from build123d import *

# Parameters (mm, degrees)
SKETCH033_W   = 68
SKETCH033_H   = 36
PAD021_DEPTH  = 1
SKETCH034_W   = 68
SKETCH034_H   = 36
SKETCH034_W_2 = 66
SKETCH034_H_2 = 34
PAD022_DEPTH  = 3
SKETCH036_R   = 1.5
PAD024_DEPTH  = 3
BOX001_W      = 70
BOX001_H      = 38
BOX001_DEPTH  = 5


with BuildPart() as bottommold:
    # Sketch033 → Pad021 (new body)
    with BuildSketch(Plane.XY):
        Rectangle(SKETCH033_W, SKETCH033_H)
    extrude(amount=PAD021_DEPTH)

    # Sketch034 (on Face6 of Pad021) → Pad022 (join)
    with BuildSketch(Plane.XY.offset(1)):
        Rectangle(SKETCH034_W, SKETCH034_H)
        Rectangle(SKETCH034_W_2, SKETCH034_H_2, mode=Mode.SUBTRACT)
    extrude(amount=PAD022_DEPTH)

    # Sketch036 → Pad024 (join)
    with BuildSketch(Plane.XY.offset(1)):
        with Locations((-31, 15)):
            Circle(SKETCH036_R)
        with Locations((31, 15)):
            Circle(SKETCH036_R)
        with Locations((-31, -15)):
            Circle(SKETCH036_R)
        with Locations((31, -15)):
            Circle(SKETCH036_R)
    extrude(amount=PAD024_DEPTH)


with BuildPart() as bottommold_1:
    # Body007 placement: moved
    add(bottommold.part.moved(Location((100, 78, 0))))


with BuildPart() as bottom_mold:
    # Box001 → Box001 (new body)
    with BuildSketch(Plane(origin=(65, 59, 0), x_dir=(1, 0, 0), z_dir=(0, 0, 1))):
        with Locations((35, 19)):
            Rectangle(BOX001_W, BOX001_H)
    extrude(amount=BOX001_DEPTH)

    # Cut001: cut BottomMold
    add(bottommold_1.part, mode=Mode.SUBTRACT)


solid = bottom_mold.part
Build history of the part. All positions in model axes, mm. A direction names the side the tool comes from. Give positions to 0.01 mm unless a question says otherwise; leave off trailing zeros. Write each loop counter-clockwise with the first axis right and the second up, starting at its lowest first coordinate (ties: lowest second). Pieces come first, ordered by that corner, then holes. Notation, with made-up numbers: (66.5, 16.5) - (80.5, 16.5) arc R29 cw to (80.5, 53.5) - close; hole circle Ø9 at (60, -16.5). An arc over 180 degrees is marked (long way). Use one line per item in the form item = value. Start each with the question number.
1. Band-saw the part on B-B on x = 93. Write the cut outline in (y, z), plus the area to 3 significant figures.
2. Probe line 1 (Y direction, x = 131, z = 3.2); line 2 (X direction, y = 74, z = 3.4); line 3 (Y direction, x = 87, z = 1.4). List the from-to ranges inside material, lowest first. Write a range as [from, to].
3. Two-plate mould, pull along Y, no slides. Class faces 1 (the face through (100, 78, 5)), 2 (the face through (100, 59, 2)), 3 (the face through (69, 93, 4)): released by +Y, released by -Y, zero draft, split by the parting line, or undercut.
4. Band-saw the part on A-A on z = 2.65. Write the cut outline in (x, y), plus the area to 3 significant figures.
5. Band-saw the part on D-D on x = 131. Write the cut outline in (y, z).
6. Drop flat-ended pins along their axis: pin 1 Ø0.9 at (x, y) = (69.5, 63.5) entering from -Z; pin 2 Ø10 at (x, y) = (79.5, 82) entering from -Z. Give the stop position or say it passes through.
7. 3-axis set-ups, long thin cutter, end or side, ignore diameter. For faces 4 (the face through (100, 97, 2)), 5 (the face through (69.806, 94.265, 2.479)): which of +Z, -Z, +X, -X, +Y, -Y reach the whole face in a straight line?
8. Band-saw the part on C-C on y = 93. Write the cut outline in (x, z).
Conclusion:
q1.outline = (59, 0) - (60, 0) - (60, 4) - (61, 4) - (61, 1) - (95, 1) - (95, 4) - (96, 4) - (96, 0) - (97, 0) - (97, 5) - (59, 5) - close
q1.area = 148 mm²
q2.line_1 = [59, 60], [61, 61.5], [64.5, 91.5], [94.5, 95], [96, 97]
q2.line_2 = [65, 66], [67, 133], [134, 135]
q2.line_3 = [59, 60], [61, 95], [96, 97]
q3.face_1 = zero draft
q3.face_2 = released by -Y
q3.face_3 = undercut
q4.outline = (65, 59) - (135, 59) - (135, 97) - (65, 97) - close; (67, 61) - (133, 61) - (133, 95) - (67, 95) - close; hole (66, 60) - (134, 60) - (134, 96) - (66, 96) - close; hole circle Ø3 at (69, 63); hole circle Ø3 at (69, 93); hole circle Ø3 at (131, 63); hole circle Ø3 at (131, 93)
q4.area = 2,430 mm²
q5.outline = (59, 0) - (60, 0) - (60, 4) - (61, 4) - (61, 1) - (61.5, 1) - (61.5, 4) - (64.5, 4) - (64.5, 1) - (91.5, 1) - (91.5, 4) - (94.5, 4) - (94.5, 1) - (95, 1) - (95, 4) - (96, 4) - (96, 0) - (97, 0) - (97, 5) - (59, 5) - close
q6.pin_1 = 4
q6.pin_2 = 1
q7.face_4 = +Z, -Z, +X, -X, +Y
q7.face_5 = -Z
q8.outline = (65, 0) - (66, 0) - (66, 4) - (67, 4) - (67, 1) - (67.5, 1) - (67.5, 4) - (70.5, 4) - (70.5, 1) - (129.5, 1) - (129.5, 4) - (132.5, 4) - (132.5, 1) - (133, 1) - (133, 4) - (134, 4) - (134, 0) - (135, 0) - (135, 5) - (65, 5) - close
